The model under review builds one solid part; all positions refer to its coordinate system, in mm. A direction names the side the tool comes from. Round coordinates to 2 decimals unless told otherwise and drop trailing zeros. Order: outer loops, then holes, each group sorted by start corner. A loop starts at its lowest first (then second) coordinate and runs counter-clockwise, first axis right, second up. Notation, with made-up numbers: M -2,-26.75 L 36,-26.75 A20 ccw 36,5.25 Z; hole C 1,-37.5 d3. An arc over 180 degrees is marked long. Answer as a JSON object with one key per item and string values. Group by question number.
1. Add section A-A on x = 2.5. State the section outline as (y, z) points.
2. Machinability: for faces 1 (the face through (-5, 2, -32.905)), 2 (the face through (4, 1, -19)), 3 (the face through (3, 6, -19)), which of the approach directions +Z, -Z, +X, -X, +Y, -Y give a long, thin tool a straight path to every point of the face, cutting with its end or side? Answer none if there is none.
3. Clearance check with flat-ended pins moving along their axes: P1, Ø4, axis at x = -13.5, y = 4, coming from the +Z side; P2, Ø4, axis at y = 4.5, z = -17, coming from the -X side; P3, Ø4.5, axis at y = 3.5, z = -36, coming from the -X side. State where each tip first meets the part, or that it passes through.
4. To check wall thickness, follow probe 1 along X at (y, z) = (0.5, -8); probe 2 along Z at (x, y) = (-0.5, 1.75); probe 3 along Z at (x, y) = (0.25, 2). State the ranges of each line that lie inside material, in increasing order. Write a range as [from, to].
5. Add section C-C on x = -6.5. State the section outline as (y, z) points.
6. Add section B-B on z = -3. State the section outline as (x, y) points.
7. Mouldability with a two-part tool opening along X and no side actions: class faces 4 (the face through (-4, 3, -26.983)), 5 (the face through (-0.64, 0.16, -8.47)), 6 (the face through (0, 5.2, -33.6)), 7 (the face through (-2.993, 3.242, -28.498)) as released by +X, released by -X, zero draft, split by the parting line, or undercut.
Autodesk Inventor part; units mm, degrees
ref_plane "Work Plane1" through (4.3209, 10, 0) normal (0, 1, 0) x (1, 0, 0)
ref_plane "YZ Plane" through (0, 0, 0) normal (1, 0, 0) x (0, 1, 0)
ref_plane "XZ Plane" through (0, 0, 0) normal (0, 1, 0) x (-1, 0, 0)
sketch "Sketch2" plane through (0, 0, 0) normal (0, 1, 0) x (-1, 0, 0)
  line L0 (0, 0) -> (23.273, 0)
  line L1 (23.273, 0) -> (23.273, -37.9053)
  line L2 (23.273, -37.9053) -> (0, -37.9053)
  line L3 (0, -37.9053) -> (0, 0)
  line L4 (26.75, 0) -> (-5, 0)
  line L5 (-5, 0) -> (-5, -37.9053)
  line L6 (-5, -37.9053) -> (26.75, -37.9053)
  line L7 (26.75, -37.9053) -> (26.75, 0)
  point P0 (0, -37.9053)
  dimension "d21" = 37.9053
  dimension "d22" = 23.273
  dimension "d36" = 5
  dimension "d37" = 31.75
extrude "Extrusion1" add sketch "Sketch2" along normal blind 10
sketch "Sketch6" plane through (-26.75, 0, 0) normal (0, 0, 1) x (1, 0, 0)
  line L0 (31.75, 0) -> (31.75, 10)
  line L1 (31.75, 0) -> (31.75, 10)
  line L2 (31.75, 0) -> (0, 0)
  line L3 (30.3918, 0) -> (30.3918, 10)
  line L4 (31.75, 10) -> (0, 10)
  line L5 (30.3918, 10) -> (55.3918, 10) construction
  line L6 (0, 0) -> (0, 10)
  line L7 (0, 0) -> (0, 0.5)
  line L8 (30.3918, 10) -> (7.0432, 0)
  point P0 (26.75, 0)
  dimension "d38" = 1.3582
  dimension "d41" = 0.5
  dimension "d96" = 25.4
  dimension "d97" = 66.815
extrude "Extrusion2" cut sketch "Sketch6" against normal up to surface (37.9053 mm away) contours L8 L2 L6 L4
sketch "Sketch8" plane through (0, 0, 0) normal (0, -1, 0) x (1, 0, 0)
  line L0 (-26.75, -37.9053) -> (-26.75, 0)
  line L1 (-26.75, -10.922) -> (3, -10.922)
  line L2 (3, -10.922) -> (3, -26.9833)
  line L3 (3, -26.9833) -> (-26.75, -26.9833)
  line L4 (-26.75, -26.9833) -> (-26.75, -10.922)
  line L5 (-26.75, 0) -> (5, 0)
  line L6 (5, -37.9053) -> (-26.75, -37.9053)
  line L7 (5, 0) -> (5, -37.9053)
  point P0 (0, 0)
  point P1 (-26.75, -26.9833)
  dimension "d44" = 10.922
  dimension "d45" = 10.922
  dimension "d46" = 2
extrude "Extrusion3" cut sketch "Sketch8" against normal blind 25.4 contours L0 L1 L2 L3
ref_plane "Work Plane1" through (4.3209, 10, 0) normal (0, 1, 0) x (1, 0, 0)
sketch "Sketch12" plane through (0, 0, 0) normal (0, -1, 0) x (1, 0, 0)
  line L0 (3.6418, 0) -> (-26.75, 0)
  line L1 (-26.75, 0) -> (0, 0)
  line L2 (0, 0) -> (0, -5)
  line L3 (0, -5) -> (-26.75, -5)
  line L4 (-26.75, -5) -> (-26.75, 0)
  line L5 (-26.75, -37.9053) -> (0, -37.9053)
  line L6 (0, -37.9053) -> (0, -32.9053)
  line L7 (0, -32.9053) -> (-26.75, -32.9053)
  line L8 (-26.75, -32.9053) -> (-26.75, -37.9053)
  line L9 (5, 0) -> (0, 0)
  line L10 (0, 0) -> (0, -1)
  line L11 (0, -1) -> (5, -1)
  line L12 (5, -1) -> (5, 0)
  line L13 (5, 0) -> (5, -37.9053)
  line L14 (5, -37.9053) -> (0, -37.9053)
  line L15 (0, -37.9053) -> (0, -36.9053)
  line L16 (0, -36.9053) -> (5, -36.9053)
  line L17 (5, -36.9053) -> (5, -37.9053)
  line L18 (5, -37.9053) -> (-26.75, -37.9053)
  point P0 (0, -37.9053)
  dimension "d69" = 5
  dimension "d70" = 5
  dimension "d73" = 1
  dimension "d74" = 1
  dimension "d75" = 0
extrude "Extrusion6" cut sketch "Sketch12" along normal through all both and the other way through all
sketch "Sketch13" plane through (0, 0, -36.9053) normal (-1, 0, 0) x (0, 0, 1)
  circle A0 centre (2, 3.9204) radius 1.5
  circle A1 centre (33.9053, 3.9204) radius 1.5
  line L0 (35.9053, 0) -> (31.9053, 0)
  line L1 (31.9053, 7.8408) -> (35.9053, 7.8408)
  line L2 (35.9053, 8.4402) -> (35.9053, 0)
  line L3 (31.9053, 2) -> (31.9053, 7.8408)
  line L4 (0, 0) -> (0, 8.4402)
  line L5 (0, 7.8408) -> (4, 7.8408)
  line L6 (4, 0) -> (0, 0)
  point P0 (36.9053, 0)
  point P1 (35.9053, 8.636)
  point P2 (0, 8.636)
  dimension "d80" = 3
  dimension "d81" = 3
  dimension "d82" = 7.8408
  dimension "d83" = 3.9204
  dimension "d84" = 4
  dimension "d85" = 2
  dimension "d86" = 2
  dimension "d87" = 3.9204
  dimension "d88" = 31.9053
  dimension "d148" = 3.9204
extrude "Extrusion7" cut sketch "Sketch13" against normal blind 25.4
sketch "Sketch15" plane through (3, 9.7251, -10.922) normal (-0.3937008, 0.9192386, 0) x (0.9192386, 0.3937008, 0)
  circle A0 centre (-20.2819, -2.4315) radius 1.1146
  circle A1 centre (-7.7426, 18.5871) radius 1.229
  line L0 (-20.2819, -2.4315) -> (-20.2819, 18.5871)
  line L1 (-20.2819, 18.5871) -> (-7.7426, 18.5871)
  line L2 (-7.7426, 18.5871) -> (-7.7426, -2.4315)
  line L3 (-7.7426, -2.4315) -> (-20.2819, -2.4315)
  line L4 (-12.8147, 2.62) -> (-12.8147, 13.4413)
  line L5 (-12.8147, 13.4413) -> (-2.3681, 13.4413)
  line L6 (-2.3681, 13.4413) -> (-2.3681, 2.62)
  line L7 (-2.3681, 2.62) -> (-12.8147, 2.62)
  line L8 (-22.0533, -4.4694) -> (-22.0533, 20.5306)
  line L9 (-22.0533, 20.5306) -> (1.9467, 20.5306)
  line L10 (1.9467, 20.5306) -> (1.9467, -4.4694)
  line L11 (1.9467, -4.4694) -> (-22.0533, -4.4694)
  line L12 (-3.2636, 21.9833) -> (-24.7018, 21.9833)
  line L13 (-24.7018, -5.922) -> (-3.2636, -5.922)
  circle A2 centre (-20.2819, 18.5871) radius 1.1245
  line L14 (0, 16.0613) -> (0, 0)
  line L15 (1.9467, -9.922) -> (1.9467, 25.9833)
  circle A3 centre (-7.7426, -2.4315) radius 1.1245
  point P0 (-6.5865, -10.922)
  dimension "d107" = 21.0186
  dimension "d108" = 12.5392
  dimension "d110" = 25
  dimension "d111" = 24
  dimension "d112" = 4.3148
  dimension "d113" = 9.2386
  dimension "d114" = 7.0893
  dimension "d115" = 7.0893
  dimension "d117" = 1.9436
  dimension "d118" = 2.0378
  dimension "d119" = 1.7714
  dimension "d120" = 9.6893
  dimension "d122" = 1.4526
  dimension "d123" = 1.4526
  dimension "d124" = 2.249
  dimension "d133" = 0
  dimension "d134" = 2.249
hole "Hole3" at (-15.6439, 1.7401, -8.4905) at (-4.1173, 6.6768, -8.4905) at (-4.1173, 6.6768, -29.5091) at (-15.6439, 1.7401, -29.5091) direction (0.3937008, -0.9192386, 0) diameter 2.1211 depth 7.1 tip angle 118 countersink diameter 2.125 countersink angle 90
chamfer "Chamfer3" distance 2 distance2 2 1 edges at (3, 0, -18.9526) measured on face at (4.3333, 0, -21.6295)
equation "\"d83\" = 0.5 * d82"
equation "\"d85\" = 0.5 * d84"
equation "\"d86\" = d85"
equation "\"d87\" = d83"
equation "\"d115\" = d114"
equation "\"d122\" = d123"
properties part number "Camera Angle"
Recorded:
{
 "1": {"outline": "M 0,-36.91 L 9.51,-36.91 L 9.51,-26.98 L 0,-26.98 Z; M 0,-10.92 L 9.51,-10.92 L 9.51,-1 L 0,-1 Z; hole C 3.92,-34.91 d3; hole C 3.92,-3 d3"},
 "2": {"face 1": "-Z, -X, +Y, -Y", "face 2": "-X, -Y", "face 3": "-X, +Y, -Y"},
 "3": {"P1": "stops at z = -5", "P2": "stops at x = 3", "P3": "stops at x = 0"},
 "4": {"probe 1": "x = [-18.54, -16.14], [-14.09, -2.49], [-0.47, 5]", "probe 2": "z = [-32.91, -26.98], [-10.92, -5]", "probe 3": "z = [-36.91, -26.98], [-10.92, -1]"},
 "5": {"outline": "M 0,-32.91 L 5.66,-32.91 L 5.66,-26.98 L 0,-26.98 Z; M 0,-10.92 L 5.66,-10.92 L 5.66,-5 L 0,-5 Z"},
 "6": {"outline": "M 0,0 L 5,0 L 5,2.42 L 0,2.42 Z; M 0,5.42 L 5,5.42 L 5,10 L 3.64,10 L 0,8.44 Z"},
 "7": {"face 4": "zero draft", "face 5": "undercut", "face 6": "released by -X", "face 7": "undercut"}
}
